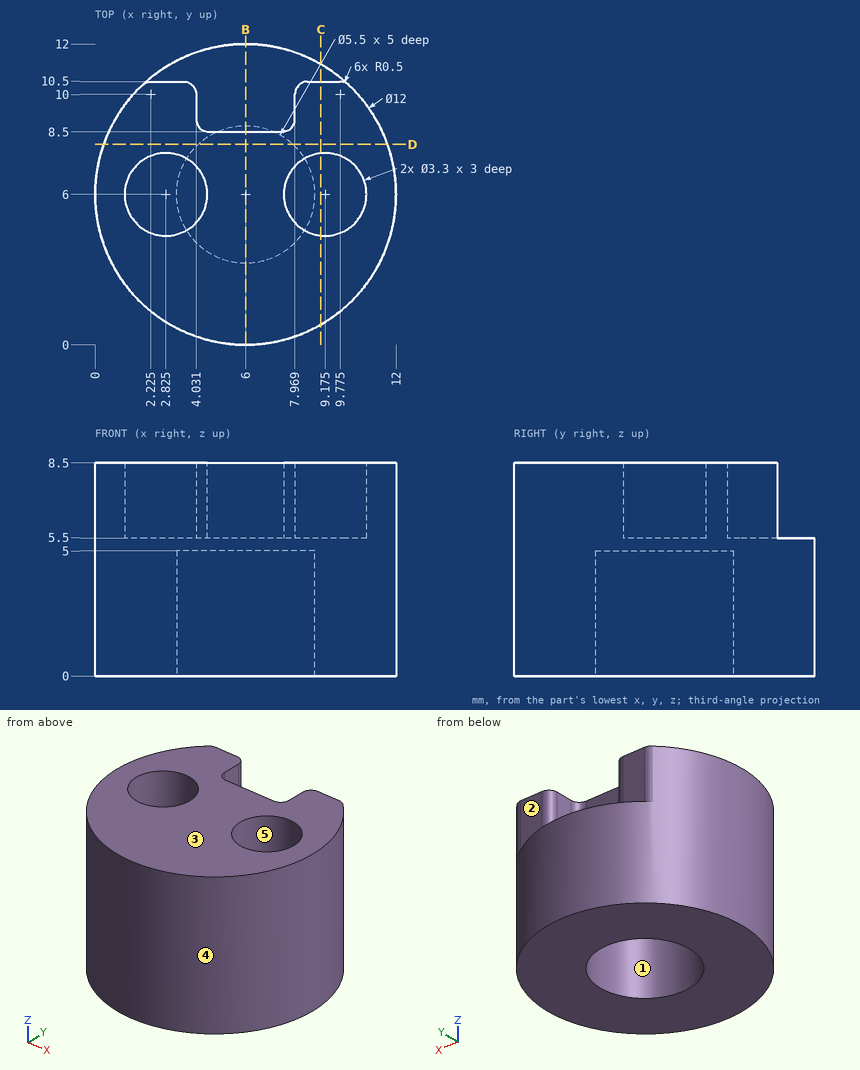
Answer from the drawing. Dimensions are ordinates in mm from the lowest x, y and z of the part. A direction names the side the tool comes from. Give positions to 0.01 mm unless a question says otherwise; leave off trailing zeros. Write each loop counter-clockwise with the first axis right and the second up, starting at its lowest first coordinate (ties: lowest second). Pieces come first, ordered by that corner, then holes. Notation, with made-up numbers: (48.5, -25) - (61.5, -25) arc R8 ccw to (61.5, -18) - close; hole circle Ø3 at (28.25, 56). An arc over 180 degrees is marked (long way). One line per item, written item: value. Start each with the question number.
1. For the marked faces 1, 2, 3, 4 and 5, determine the directions among +Z, -Z, +X, -X, +Y, -Y from which every point of the face is accessible in a straight line to the end or side of a thin tool.
2. Find section B-B (x = 6). Write down the section's boundary in (y, z), then the cut area to 3 significant figures.
3. Find section D-D (y = 8). Write down the section's boundary in (x, z), then the cut area to 3 significant figures.
4. Consider probe 1 along X at (y, z) = (6, 1.4); probe 2 along X at (y, z) = (7.25, 8.25). Determine where each line is inside the solid, lowest interval first.
5. Find section C-C (x = 9). Write down the section's boundary in (y, z).
6. Given pin 1 (1.5 mm diameter, centred on x = 2.5, z = 7, fed in from +Y); pin 2 (1 mm diameter, centred on y = 10.5, z = 7, fed in from +X); pin 3 (3 mm diameter, centred on x = 9, z = 4.5, fed in from +Y), each flat-ended and moving along its own axis, determine where each tip first touches the part or whether it passes through.
Geometry results:
1. face 1: -Z
1. face 2: +Z, +X, -X, +Y
1. face 3: +Z, +X, -X, +Y, -Y
1. face 4: +Z, -Z
1. face 5: +Z
2. outline: (0, 0) - (3.25, 0) - (3.25, 5) - (8.75, 5) - (8.75, 0) - (12, 0) - (12, 5.5) - (8.5, 5.5) - (8.5, 8.5) - (0, 8.5) - close
2. area: 64.0 mm2
3. outline: (0.34, 0) - (4.11, 0) - (4.11, 5) - (7.89, 5) - (7.89, 0) - (11.66, 0) - (11.66, 8.5) - (0.34, 8.5) - close
3. area: 77.3 mm2
4. probe 1: 0 to 3.25, 8.75 to 12
4. probe 2: 0.13 to 1.75, 3.9 to 8.1, 10.25 to 11.87
5. outline: (0.8, 0) - (11.2, 0) - (11.2, 5.5) - (10.5, 5.5) - (10.5, 8.5) - (7.64, 8.5) - (7.64, 5.5) - (4.36, 5.5) - (4.36, 8.5) - (0.8, 8.5) - close
6. pin 1: y = 10.5
6. pin 2: x = 10.47
6. pin 3: y = 11.81
